Geometry: see drawing. Coordinates: mm, zero at the bounding-box minimum. A direction names the side the tool comes from. Give positions to 0.01 mm unless a question says otherwise; leave off trailing zeros. Loops run counter-clockwise (first coordinate to the right, second up) from the corner with the lowest first, then second, coordinate; pieces in that order, holes last. Notation, with made-up numbers: M -33,78.25 L -18,78.25 A30 ccw -18,106.25 Z; hole C 50.25,-4.75 d9. An arc over 180 degrees is marked long. Put each result on its own line as item: value.
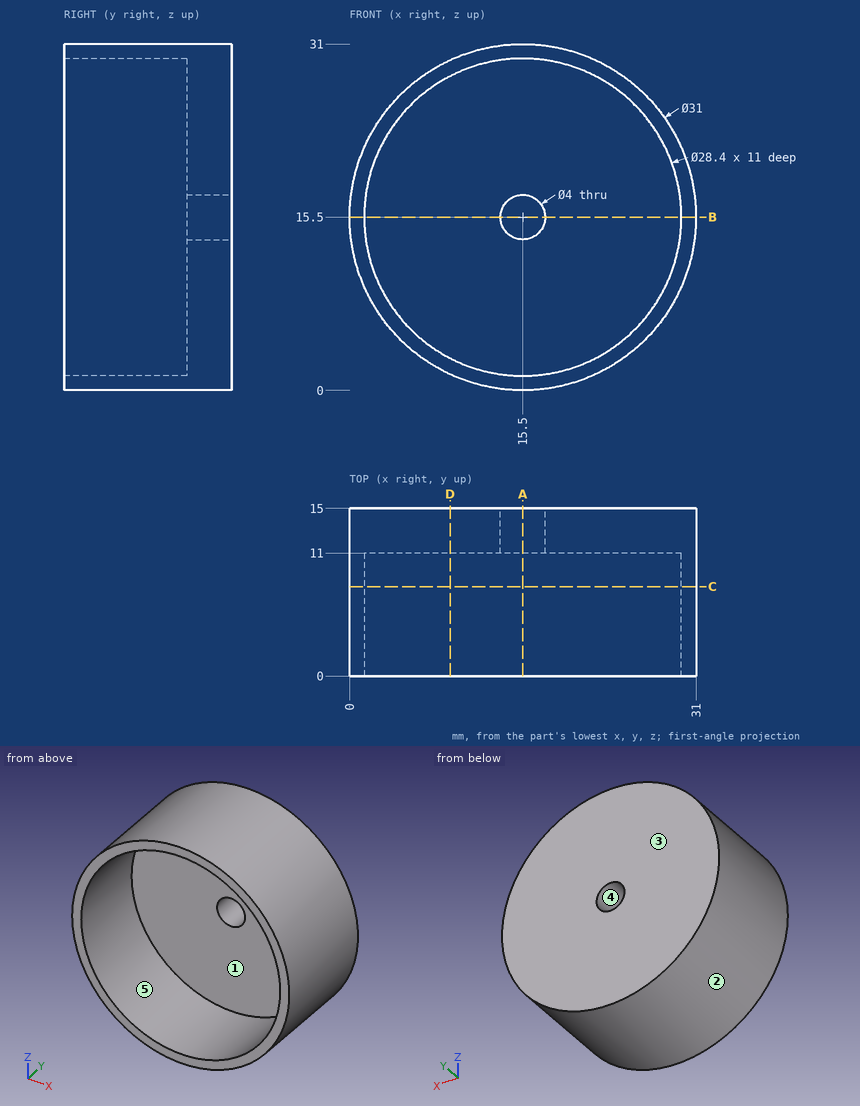
Item 1: Mould query, pull axis Z, two halves, no side actions, for the marked faces 1, 2 and 3. Classes: pulls with the +Z half, pulls with the -Z half, needs draft (parallel to the pull), parting line crosses it, or undercut.
Output values:
face 1: undercut
face 2: parting line crosses it
face 3: needs draft
Item 2: Pin query (flat end, axial travel): pin 1 Ø3 at (x, z) = (12, 21.5) entering from -Y; pin 2 Ø8 at (x, y) = (16.5, 4.5) entering from +Z; pin 3 Ø6 at (x, y) = (27.5, 10) entering from +Z. Return the tip coordinate at first contact, or that it passes through.
Output values:
pin 1: y = 11
pin 2: z = 31
pin 3: z = 28.12
Item 3: Line query: probe 1 along Z at (x, y) = (15.5, 3.25); probe 2 along Z at (x, y) = (15.5, 12.9); probe 3 along Y at (x, z) = (6, 6). Output: solid intervals per line, ascending. Write a range as [from, to].
Output values:
probe 1: [0, 1.3], [29.7, 31]
probe 2: [0, 13.5], [17.5, 31]
probe 3: [11, 15]
Item 4: Section B-B on z = 15.5. Output: boundary loops of the cut face in (x, y), then the cut area to 3 significant figures.
Output values:
outline: M 0,0 L 1.3,0 L 1.3,11 L 13.5,11 L 13.5,15 L 0,15 Z; M 17.5,11 L 29.7,11 L 29.7,0 L 31,0 L 31,15 L 17.5,15 Z
area: 137 mm²
Item 5: Section D-D on x = 9. Output: boundary loops of the cut face in (y, z), then the cut area to 3 significant figures.
Output values:
outline: M 0,1.43 L 15,1.43 L 15,29.57 L 0,29.57 L 0,28.12 L 11,28.12 L 11,2.88 L 0,2.88 Z
area: 144 mm²
Item 6: Set-up query: the marked faces 4 and 5. Return all of +Z, -Z, +X, -X, +Y, -Y with unobstructed straight access to the full face (end or side cutting, diameter ignored); none if empty.
Output values:
face 4: +Y, -Y
face 5: -Y
Item 7: Section C-C on y = 8. Output: boundary loops of the cut face in (x, z).
Output values:
outline: C 15.5,15.5 d31; hole C 15.5,15.5 d28.4
Item 8: Section A-A on x = 15.5. Output: boundary loops of the cut face in (y, z).
Output values:
outline: M 0,0 L 15,0 L 15,13.5 L 11,13.5 L 11,1.3 L 0,1.3 Z; M 0,29.7 L 11,29.7 L 11,17.5 L 15,17.5 L 15,31 L 0,31 Z
